Work out the finished part from the listing and answer in its coordinate system (mm). A direction names the side the tool comes from. Coordinates: 2 decimals unless noted, no trailing zeros. Write each loop counter-clockwise with the first axis right and the second up, starting at its lowest first coordinate (ties: lowest second). Pieces come first, ordered by that corner, then holes. Notation, with made-up numbers: (-5.75, 80) - (21.25, 80) arc R8 cw to (21.25, 92) - close; hole circle Ø2 at (-13, 81). An arc over 180 degrees is marked (long way). Use a Markdown table: item, result. Add a question column.
(1) Find the intervals of material crossed by line 1 (Z direction, x = 0, y = -3) (3 decimals); line 2 (Y direction, x = -5, z = 0.5); line 3 (Y direction, x = -2, z = 4), in increasing order. Write a range as from..to.
(2) The part is cut by section D-D, the plane z = 2. Give the vertices of the cut face in (x, y), then the cut area to 3 significant figures.
(3) The part is cut by section B-B, the plane y = -6.5. Give the vertices of the cut face in (x, z) (3 decimals), then the cut area to 3 significant figures.
(4) The part is cut by section C-C, the plane y = -1.5. Give the vertices of the cut face in (x, z) (3 decimals).
(5) A tool of negligible diameter and unlimited length cuts with its end or side. For faces 1 (the face through (-4.243, -18, 0)), 2 (the face through (4.243, -18, 0)), 3 (the face through (0.59, -12.04, 4.46)), 4 (the face through (-3.943, -18, 0)), 5 (the face through (1.2, -10, 0)), from which of +Z, -Z, +X, -X, +Y, -Y can it reach the whole face along a straight path? Write none if from no direction.
(6) Given pin 1 Ø5 at (x, y) = (0, -2) entering from -Z (3 decimals); pin 2 Ø0.9 at (x, y) = (0, -18) entering from -Z; pin 3 Ø3.5 at (x, y) = (-0.5, -18) entering from +Z; pin 4 Ø6 at (x, z) = (-3, -2.5) entering from +Y, each flat-ended and moving along its own axis, determine where each tip first touches the part or whether it passes through.
(7) The part is cut by section A-A, the plane y = -15.75. Give the vertices of the cut face in (x, z).
(8) For a pull along Z with two mould halves and no side action, classify faces 6 (the face through (3.943, -18, 0)), 7 (the face through (0.37, -4.93, 2.85)), 8 (the face through (0.504, -3.042, 3.842)), 9 (the face through (0, -18, -3.943)) as released by +Z, released by -Z, zero draft, split by the parting line, or undercut.
from build123d import *

# Parameters (mm, degrees)
SKIZZE2_W                       = 0.3
SKIZZE2_H                       = 3
SKIZZE2_W_2                     = 3
SKIZZE2_H_2                     = 0.3
AUFSATZ_LINEAR_AUSTRAGEN1_DEPTH = 6
VERRUNDUNG1_R                   = 0.75


with BuildPart() as part:
    # Skizze1 → Rotation1 (revolve)
    with BuildSketch(Plane.XY):
        Polygon((-3.875, 0), (-3.875, -6), (-5.5, -6), (-5.5, -9), (-4.5, -9), (-4.5, -15), (0, -15), (0, -2.3), (-1, -2.3), (-1, -10), (-2.875, -10), (-2.875, 0), align=None)
    revolve(axis=Axis((0, -15, 0), (0, 1, 0)))

    # Skizze2 → Aufsatz-Linear austragen1 (add)
    with BuildSketch(Plane.XZ.offset(15)):
        with Locations((-4.092640687, 0)):
            Rectangle(SKIZZE2_W, SKIZZE2_H)
        with Locations((4.092640687, 0)):
            Rectangle(SKIZZE2_W, SKIZZE2_H)
        with Locations((0, -4.092640687)):
            Rectangle(SKIZZE2_W_2, SKIZZE2_H_2)
    extrude(amount=AUFSATZ_LINEAR_AUSTRAGEN1_DEPTH)

    # Verrundung1
    verrundung1_edges = [part.edges().sort_by_distance(p)[0] for p in [
        (1, -2.3, 0),
    ]]
    fillet(verrundung1_edges, radius=VERRUNDUNG1_R)


solid = part.part
Model answer:
| question | item | result |
|---|---|---|
| 1 | line 1 | -3.875..-2.875, -0.998..0.998, 2.875..3.875 |
| 1 | line 2 | -9..-6 |
| 1 | line 3 | -15..-6 |
| 2 | outline | (-5.12, -9) - (-4.03, -9) - (-4.03, -15) - (4.03, -15) - (4.03, -9) - (5.12, -9) - (5.12, -6) - (3.32, -6) - (3.32, 0) - (2.07, 0) - (2.07, -10) - (-2.07, -10) - (-2.07, 0) - (-3.32, 0) - (-3.32, -6) - (-5.12, -6) - close |
| 2 | area | 77.6 mm^2 |
| 3 | outline | circle Ø11 at (0, 0); circle Ø2 at (0, 0); hole circle Ø5.75 at (0, 0) |
| 3 | area | 72.2 mm^2 |
| 4 | outline | circle Ø7.75 at (0, 0); hole circle Ø5.75 at (0, 0) |
| 5 | face 1 | +Z, -Z, -X, -Y |
| 5 | face 2 | +Z, -Z, +X, -Y |
| 5 | face 3 | -Y |
| 5 | face 4 | +Z, -Z, -Y |
| 5 | face 5 | +Y |
| 6 | pin 1 | z = -3.875 |
| 6 | pin 2 | z = -4.24 |
| 6 | pin 3 | z = -3.94 |
| 6 | pin 4 | y = 0 |
| 7 | outline | (-4.24, -1.5) - (-3.94, -1.5) - (-3.94, 1.5) - (-4.24, 1.5) - close; (-1.5, -4.24) - (1.5, -4.24) - (1.5, -3.94) - (-1.5, -3.94) - close; (3.94, -1.5) - (4.24, -1.5) - (4.24, 1.5) - (3.94, 1.5) - close |
| 8 | face 6 | zero draft |
| 8 | face 7 | undercut |
| 8 | face 8 | split by the parting line |
| 8 | face 9 | released by +Z |
